Geometry check sheet. Reference: drawing and pictorial views, mm from the part's lowest x, y, z. A direction names the side the tool comes from. Round coordinates to 2 decimals unless told otherwise and drop trailing zeros. Write each loop counter-clockwise with the first axis right and the second up, starting at its lowest first coordinate (ties: lowest second). Pieces come first, ordered by that corner, then holes. Notation, with made-up numbers: (2, 61) -> (40, 61) arc R23 ccw to (40, 93) -> close; hole circle Ø8 at (33, 45.25). An arc over 180 degrees is marked (long way). Answer as a JSON object with one key per item and string values. Group by question number.
(1) Sectioned sample at C-C on z = 44. Record the cut outline in (x, y).
(2) Scan lines: L1, parallel to X at y = 42, z = 53; L2, parallel to X at y = 11, z = 22; L3, parallel to Y at x = 27.5, z = 6.5. Record each from-to range of solid material in increasing order. Write a range as from..to.
(3) Sectioned sample at B-B on z = 28.5. Record the cut outline in (x, y), and give its area (3 significant figures).
(4) Set-up check for the marked faces 1, 2, 3 and 4: record each of +Z, -Z, +X, -X, +Y, -Y from which the full face is reachable in a straight line by a thin tool's end or side.
(5) Draft check along X on the marked faces 5, 6 and 7. Enter one of: released by +X, released by -X, zero draft, split by the parting line, or undercut.
(6) Sectioned sample at D-D on y = 31. Record the cut outline in (x, z).
(7) Gauge pin test, flat ends, axial feed: pin 1 Ø10 at (x, y) = (25, 10.5) entering from -Z; pin 2 Ø9 at (x, y) = (76.5, 34.5) entering from -Z; pin 3 Ø22 at (y, z) = (7.5, 14.5) entering from +X; pin 4 Ø18 at (x, z) = (38, 20) entering from +Y. Record the tip position at first contact, or that the pin passes through.
(8) Sectioned sample at A-A on x = 69. Record the cut outline in (y, z).
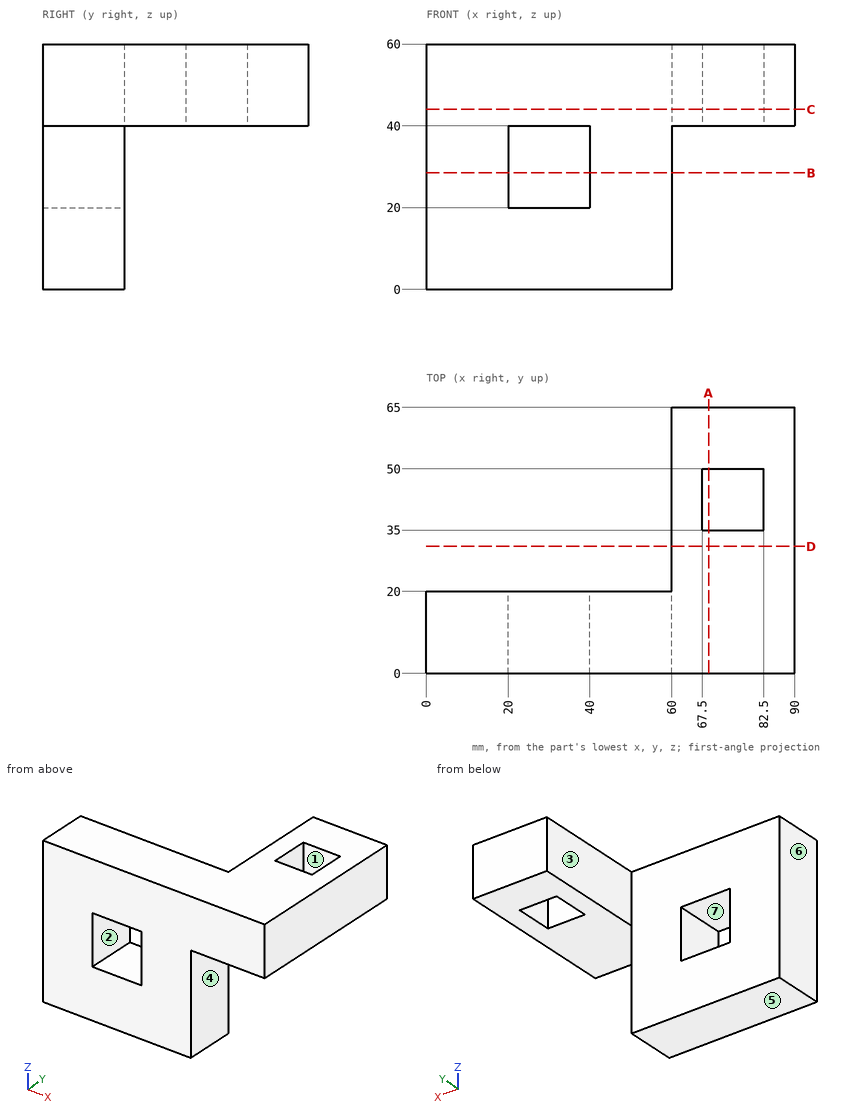
Computed values:
{
 "1": {"outline": "(0, 0) -> (90, 0) -> (90, 65) -> (60, 65) -> (60, 20) -> (0, 20) -> close; hole (67.5, 35) -> (82.5, 35) -> (82.5, 50) -> (67.5, 50) -> close"},
 "2": {"L1": "60..67.5, 82.5..90", "L2": "0..20, 40..60", "L3": "0..20"},
 "3": {"outline": "(0, 0) -> (20, 0) -> (20, 20) -> (0, 20) -> close; (40, 0) -> (60, 0) -> (60, 20) -> (40, 20) -> close", "area": "800 mm2"},
 "4": {"face 1": "+Z, -Z", "face 2": "+Y, -Y", "face 3": "+Z, -Z, -X, +Y", "face 4": "-Z, +X, +Y, -Y"},
 "5": {"face 5": "zero draft", "face 6": "released by -X", "face 7": "undercut"},
 "6": {"outline": "(60, 40) -> (90, 40) -> (90, 60) -> (60, 60) -> close"},
 "7": {"pin 1": "z = 0", "pin 2": "z = 40", "pin 3": "x = 60", "pin 4": "y = 20"},
 "8": {"outline": "(0, 40) -> (35, 40) -> (35, 60) -> (0, 60) -> close; (50, 40) -> (65, 40) -> (65, 60) -> (50, 60) -> close"}
}
